Input: dimensioned drawing with shaded views. Units: mm. Origin: part minimum x, y, z. Coordinates: 2 decimals unless noted, no trailing zeros. Order: outer loops, then holes, each group sorted by start corner. A loop starts at its lowest first (then second) coordinate and runs counter-clockwise, first axis right, second up. Notation, with made-up numbers: (30, -37.5) - (81, -37.5) arc R21 cw to (81, -1.5) - close; hole circle Ø10 at (-5, 34.25). An arc over 180 degrees is marked (long way). Answer as CSV lines item,"result". Start each with the question number.
Item 1: Section B-B (z = 37). Output: boundary loops of the cut face in (x, y).
Item 2: First-contact query: pin 1 (6 mm diameter, centred on x = 9.5, z = 45, fed in from +Y) (1 decimal); pin 2 (10 mm diameter, centred on x = 58.5, z = 47.5, fed in from -Y); pin 3 (4 mm diameter, centred on y = 66.5, z = 8, fed in from +X). Flat tips, straight axial feed; report the tip coordinate or a pass-through.
Item 3: Section A-A (z = 49.5). Output: boundary loops of the cut face in (x, y), and give its area (3 significant figures).
Item 4: Material intervals for line 1 along Z through (x, y) = (5, 33); line 2 along Y through (x, z) = (32, 24.5) (1 decimal); line 3 along Y through (x, z) = (34, 39) (1 decimal), sorted ascending.
Item 5: Draft query along X for the marked faces 1, 2 and 3. Return one class per face: +X half, -X half, draft (parallel to the pull), parting line (faces both ways), or undercut.
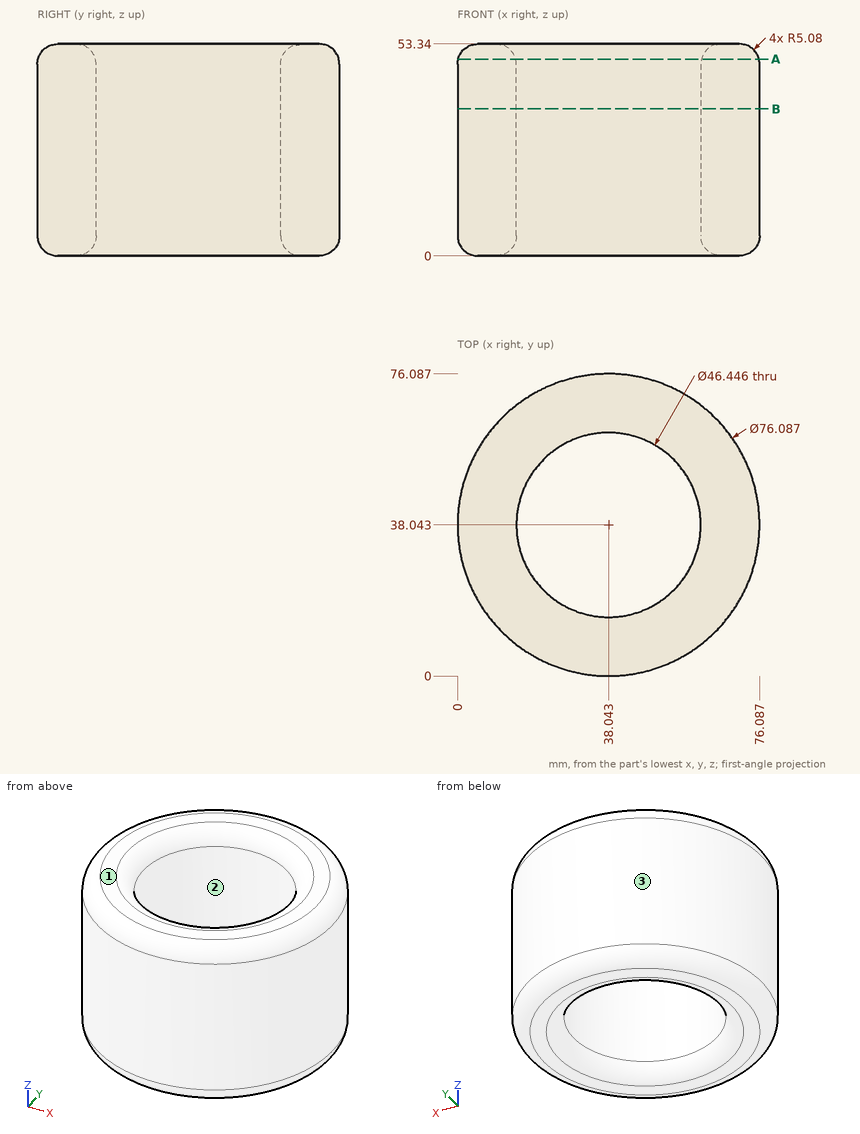
Determined:
1,outline,"circle Ø76.09 at (38.04, 38.04); hole circle Ø46.45 at (38.04, 38.04)"
2,pin 1,"stops at y = 66.2"
2,pin 2,"stops at y = 3.28"
2,pin 3,"stops at x = 65.38"
3,outline,"circle Ø75.78 at (38.04, 38.04); hole circle Ø46.75 at (38.04, 38.04)"
3,area,"2,790 mm^2"
4,line 1,"z = 0.02 to 53.32"
4,line 2,"y = 0.5 to 15.6, 60.5 to 75.6"
4,line 3,"y = 0.2 to 15.2, 60.9 to 75.9"
5,face 1,"draft"
5,face 2,"undercut"
5,face 3,"parting line"
